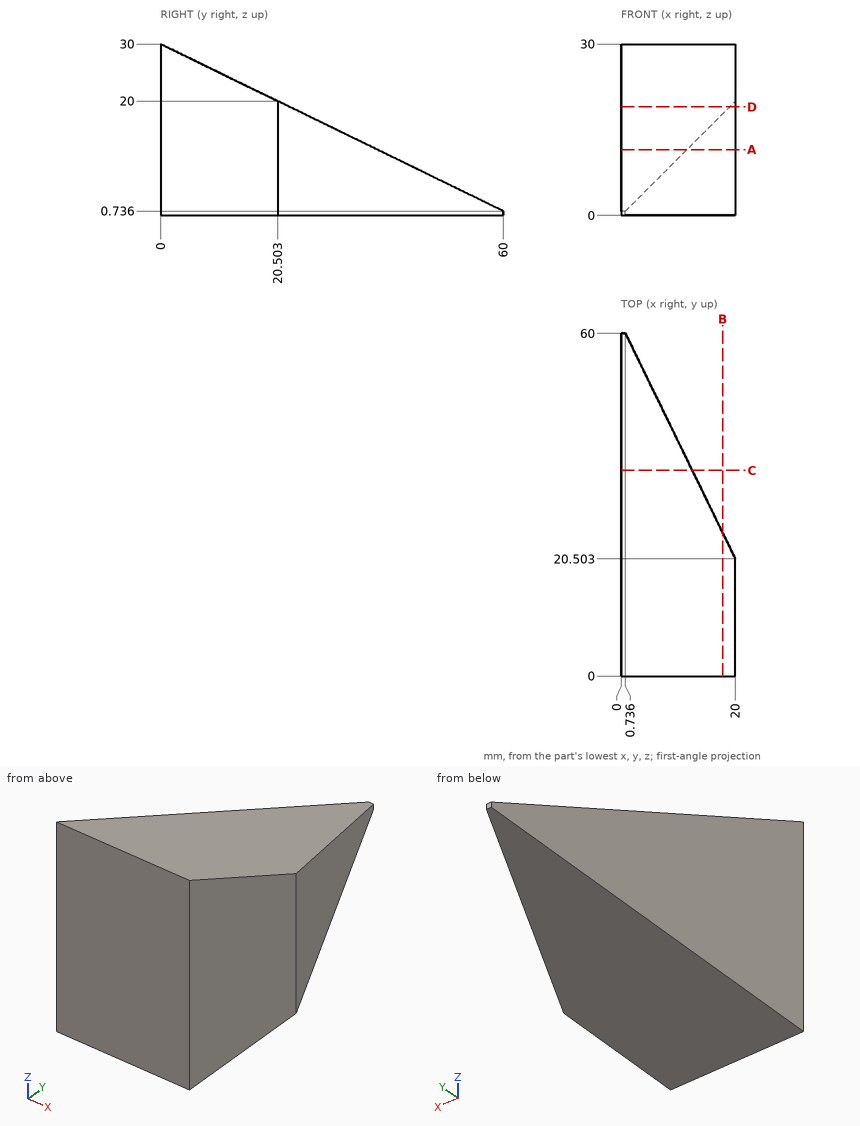
Check sheet for the drawn part. Datum: minimum x, y, z corner. Units: mm. Round coordinates to 2 decimals unless told otherwise and drop trailing zeros. Order: outer loops, then holes, each group sorted by start corner. A loop starts at its lowest first (then second) coordinate and runs counter-clockwise, first axis right, second up. Notation, with made-up numbers: (-39.5, 73.5) - (19.5, 73.5) arc R24 ccw to (19.5, 100.5) - close; hole circle Ø8 at (50.25, 16). An arc over 180 degrees is marked (long way). Use a Markdown table: item, result. Add a question column.
(1) Depth check by flat-ended pin: pin 1 (10 mm diameter, centred on x = 10.5, z = 23, fed in from +Y); pin 2 (5 mm diameter, centred on y = 30, z = 18, fed in from +X); pin 3 (1.5 mm diameter, centred on x = 14.5, y = 23.5, fed in from +Z); pin 4 (6 mm diameter, centred on y = 49.5, z = 11.5, fed in from -X). Enter the tip coordinate at first touch or a pass-through.
(2) Sectioned sample at C-C, the plane y = 36. Enter the section's corners in (x, z).
(3) Sectioned sample at D-D, the plane z = 19. Enter the section's corners in (x, y), and give its area (3 significant figures).
(4) Material ranges on line 1 along Z through (x, y) = (17, 19.5); line 2 along Y through (x, z) = (1.5, 23.25); line 3 along Z through (x, y) = (12, 35.5), recorded low to high. Write a range as [from, to].
(5) Sectioned sample at A-A, the plane z = 11.5. Enter the section's corners in (x, y), and give its area (3 significant figures).
(6) Sectioned sample at B-B, the plane x = 17.75. Enter the section's corners in (y, z).
Answers below:
| question | item | result |
|---|---|---|
| 1 | pin 1 | y = 24.6 |
| 1 | pin 2 | x = 16.23 |
| 1 | pin 3 | z = 18.9 |
| 1 | pin 4 | through |
| 2 | outline | (0, 0) - (12.44, 0) - (12.44, 12.44) - (0, 12.44) - close |
| 3 | outline | (0, 0) - (20, 0) - (20, 20.5) - (19, 22.55) - (0, 22.55) - close |
| 3 | area | 450 mm² |
| 4 | line 1 | [0, 20.49] |
| 4 | line 2 | [0, 13.84] |
| 4 | line 3 | [0, 12.69] |
| 5 | outline | (0, 0) - (20, 0) - (20, 20.5) - (11.5, 37.93) - (0, 37.93) - close |
| 5 | area | 685 mm² |
| 6 | outline | (0, 0) - (25.12, 0) - (25.12, 17.75) - (0, 30) - close |
